```python
from build123d import *

# Parameters (mm, degrees)
SKETCH1_W               = 200
SKETCH1_H               = 155
SKETCH1_R               = 3.38
BOSS_EXTRUDE1_DEPTH     = 6.35
M4X0_7_TAPPED_HOLE1_D   = 3.3
CUT_EXTRUDE1_DEPTH      = 127.675066607
CUT_EXTRUDE1_DEPTH_BACK = 127.675066607
SKETCH4_W               = 200
SKETCH4_H               = 9.5
FILLET1_R               = 10


with BuildPart() as part:
    # Sketch1 → Boss-Extrude1 (new body)
    with BuildSketch(Plane.XY):
        Rectangle(SKETCH1_W, SKETCH1_H)
        with Locations((-88.9, 71.7)):
            Circle(SKETCH1_R, mode=Mode.SUBTRACT)
        with Locations((88.9, 71.7)):
            Circle(SKETCH1_R, mode=Mode.SUBTRACT)
        with Locations((88.9, -55.3)):
            Circle(SKETCH1_R, mode=Mode.SUBTRACT)
        with Locations((-88.9, -55.3)):
            Circle(SKETCH1_R, mode=Mode.SUBTRACT)
    extrude(amount=BOSS_EXTRUDE1_DEPTH)

    # M4x0.7 Tapped Hole1 (through all)
    with Locations(Plane(origin=(51.961524227, -30, 0), x_dir=(-1, 0, 0), z_dir=(0, 0, -1))):
        with Locations((0, 0), (103.923048454, 0), (51.961524227, 90)):
            Hole(M4X0_7_TAPPED_HOLE1_D / 2)

    # Sketch4 → Cut-Extrude1 (cut, two sides: drawn at the far end of the back side and taken through both)
    with BuildSketch(Plane.XY.offset(6.35).offset(-CUT_EXTRUDE1_DEPTH_BACK)):
        with Locations((0, -72.75)):
            Rectangle(SKETCH4_W, SKETCH4_H)
    extrude(amount=CUT_EXTRUDE1_DEPTH + CUT_EXTRUDE1_DEPTH_BACK, mode=Mode.SUBTRACT)

    # Fillet1
    fillet1_edges = [part.edges().sort_by_distance(p)[0] for p in [
        (-100, -68, 3.175),
        (100, -68, 3.175),
        (-100, 77.5, 3.175),
        (100, 77.5, 3.175),
    ]]
    fillet(fillet1_edges, radius=FILLET1_R)


solid = part.part
```
Could you check a few things on this model? Use its own coordinates, in mm. Round coordinates to 2 decimals unless told otherwise and drop trailing zeros. Write each loop counter-clockwise with the first axis right and the second up, starting at its lowest first coordinate (ties: lowest second). Pieces come first, ordered by that corner, then holes. Notation, with made-up numbers: M 1,56 L 33,56 A6 ccw 33,63 Z; hole C 7.5,1 d5. An arc over 180 degrees is marked long. Write each question's results on one line, items separated by ' | '. Start each with the question number.
1. Thinking about a two-plate mould opening in Y: for faces 1 (the face through (-97.15, -64.99, 3.22)), 2 (the face through (-92.277, 71.849, 3.131)), 3 (the face through (96.99, 74.65, 3.22)), which applies, +Y half, -Y half, draft (parallel to the pull), parting line (faces both ways), or undercut?
2. I need wall thicknesses on L1, parallel to Y at x = -88.9, z = 3; L2, parallel to X at y = 70, z = 2.75; L3, parallel to Y at x = 0, z = 4.75. Which ranges of each line are inside material? Lowest first, please. Write a range as from..to.
3. I'm going to push flat-ended pins straight in: pin 1 Ø9 at (x, y) = (88.9, 71.7) entering from -Z; pin 2 Ø5.5 at (x, y) = (-88.9, -55.3) entering from -Z. Where does each tip first touch, or does it pass through?
4. Imagine slicing it at A-A on y = -55.3. List the corners of the cut face in (x, z) for me.
Result sheet:
1) face 1: -Y half | face 2: undercut | face 3: +Y half
2) L1: y = -68..-58.68, -51.92..68.32, 75.08..77.5 | L2: x = -99.68..-91.82, -85.98..85.98, 91.82..99.68 | L3: y = -68..58.35, 61.65..77.5
3) pin 1: stops at z = 0 | pin 2: passes through
4) outline: M -100,0 L -92.28,0 L -92.28,6.35 L -100,6.35 Z; M -85.52,0 L 85.52,0 L 85.52,6.35 L -85.52,6.35 Z; M 92.28,0 L 100,0 L 100,6.35 L 92.28,6.35 Z
